```python
from build123d import *

# Parameters (mm, degrees)
SKETCH1_W           = 38.1
SKETCH1_H           = 120.65
SKETCH1_W_2         = 177.8
SKETCH1_H_2         = 177.8
SKETCH1_R           = 14.605
BOSS_EXTRUDE1_DEPTH = 3.175
SKETCH2_R           = 3.175
CUT_EXTRUDE1_DEPTH  = 4.175
SKETCH2_3_W         = 12.7
SKETCH2_3_H         = 38.1
BOSS_EXTRUDE2_DEPTH = 63.5
SKETCH3_R           = 6.35
CUT_EXTRUDE2_DEPTH  = 108.95
CUT_EXTRUDE3_DEPTH  = 4.175


with BuildPart() as part:
    # Sketch1 → Boss-Extrude1 (new body)
    with BuildSketch(Plane.XY):
        with Locations((0, 149.225)):
            Rectangle(SKETCH1_W, SKETCH1_H)
        Rectangle(SKETCH1_W_2, SKETCH1_H_2)
        Circle(SKETCH1_R, mode=Mode.SUBTRACT)
    extrude(amount=BOSS_EXTRUDE1_DEPTH)

    # Sketch2 → Cut-Extrude1 (cut, through all)
    with BuildSketch(Plane.XY.offset(3.175)):
        with Locations((-38.494829198, 22.225)):
            Circle(SKETCH2_R)
        with Locations((38.494829198, 22.225)):
            Circle(SKETCH2_R)
        with Locations((0, -44.45)):
            Circle(SKETCH2_R)
    extrude(amount=-CUT_EXTRUDE1_DEPTH, mode=Mode.SUBTRACT)

    # Sketch2_3 → Boss-Extrude2 (add)
    with BuildSketch(Plane.XY.offset(3.175)):
        with Locations((-12.7, 190.5)):
            Rectangle(SKETCH2_3_W, SKETCH2_3_H)
        with Locations((12.7, 190.5)):
            Rectangle(SKETCH2_3_W, SKETCH2_3_H)
    extrude(amount=BOSS_EXTRUDE2_DEPTH)

    # Sketch3 → Cut-Extrude2 (cut, through all)
    with BuildSketch(Plane.ZY.offset(19.05)):
        with Locations((34.925, 190.5)):
            Circle(SKETCH3_R)
    extrude(amount=-CUT_EXTRUDE2_DEPTH, mode=Mode.SUBTRACT)

    # Sketch4 → Cut-Extrude3 (cut, through all)
    with BuildSketch(Plane.XY.offset(3.175)):
        with BuildLine():
            Line((-19.05, 53.881536726), (-19.05, 88.9))
            Line((-19.05, 88.9), (-88.9, 88.9))
            Line((-88.9, 88.9), (-88.9, -88.9))
            Line((-88.9, -88.9), (88.9, -88.9))
            Line((88.9, -88.9), (88.9, 88.9))
            Line((88.9, 88.9), (19.05, 88.9))
            Line((19.05, 88.9), (19.05, 53.881536726))
            ThreePointArc((19.05, 53.881536726), (46.6627796, 32.995567884), (57.15, 0))
            ThreePointArc((57.15, 0), (-32.995567884, -46.6627796), (-19.05, 53.881536726))
        make_face()
    extrude(amount=-CUT_EXTRUDE3_DEPTH, mode=Mode.SUBTRACT)


solid = part.part
```
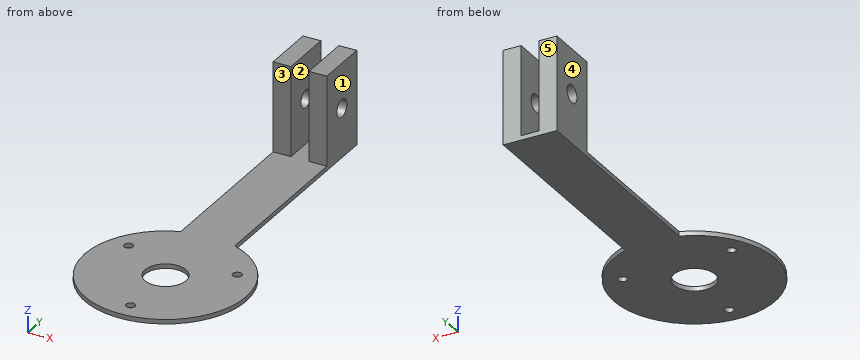
Build history of the part. All positions in model axes, mm. Face numbers are marked on the shaded views. A direction names the side the tool comes from. Coordinates: 2 decimals unless noted, no trailing zeros. Order: outer loops, then holes, each group sorted by start corner. A loop starts at its lowest first (then second) coordinate and runs counter-clockwise, first axis right, second up. Notation, with made-up numbers: (3.25, 87.25) -> (39.25, 87.25) arc R30 ccw to (39.25, 114.25) -> close; hole circle Ø1 at (52, 30). An arc over 180 degrees is marked (long way). Answer in a Markdown table with one row per item. Add a question column.
Q1. Band-saw the part on B-B, the plane x = 0. List the corners of the cut face in (y, z) (3 decimals).
Q2. Which spindle directions (+Z, -Z, +X, -X, +Y, -Y) get a long thin tool onto all of the face, cutting with end or side? Do the marked faces 1, 2, 3, 4 and 5. Say none if no direction does.
Q3. Drop flat-ended pins along their axis: pin 1 (17.5 mm diameter, centred on x = 0, y = 0, fed in from +Z); pin 2 (16.5 mm diameter, centred on y = 190.5, z = 34.925, fed in from -X); pin 3 (6.5 mm diameter, centred on x = 13.5, z = 20, fed in from -Y). Give the stop position or say it passes through.
Q4. Wall check: line 1 along Z through (x, y) = (-15, 53.5) (3 decimals); line 2 along Y through (x, z) = (9.5, 9.5). Give the ranges that are in metal, low to high. Write a range as [from, to].
Q5. Band-saw the part on D-D, the plane y = -44.45. List the corners of the cut face in (x, z) (3 decimals), then the cut area to 3 significant figures.
Q6. Band-saw the part on A-A, the plane y = 190.5. List the corners of the cut face in (x, z) (3 decimals).
Q7. Band-saw the part on C-C, the plane z = 59. List the corners of the cut face in (x, y).
Answers follow:
| question | item | result |
|---|---|---|
| 1 | outline | (-57.15, 0) -> (-47.625, 0) -> (-47.625, 3.175) -> (-57.15, 3.175) -> close; (-41.275, 0) -> (-14.605, 0) -> (-14.605, 3.175) -> (-41.275, 3.175) -> close; (14.605, 0) -> (209.55, 0) -> (209.55, 3.175) -> (14.605, 3.175) -> close |
| 2 | face 1 | +Z, -Z, +X, +Y |
| 2 | face 2 | +Z, +Y, -Y |
| 2 | face 3 | +Z, +X, -X, -Y |
| 2 | face 4 | +Z, -Z, -X, +Y |
| 2 | face 5 | +Z, -Z, +X, -X, +Y |
| 3 | pin 1 | through |
| 3 | pin 2 | x = -19.05 |
| 3 | pin 3 | y = 171.45 |
| 4 | line 1 | [0, 3.175] |
| 4 | line 2 | [171.45, 209.55] |
| 5 | outline | (-35.921, 0) -> (-3.175, 0) -> (-3.175, 3.175) -> (-35.921, 3.175) -> close; (3.175, 0) -> (35.921, 0) -> (35.921, 3.175) -> (3.175, 3.175) -> close |
| 5 | area | 208 mm^2 |
| 6 | outline | (-19.05, 0) -> (19.05, 0) -> (19.05, 28.575) -> (6.35, 28.575) -> (6.35, 3.175) -> (-6.35, 3.175) -> (-6.35, 28.575) -> (-19.05, 28.575) -> close; (-19.05, 41.275) -> (-6.35, 41.275) -> (-6.35, 66.675) -> (-19.05, 66.675) -> close; (6.35, 41.275) -> (19.05, 41.275) -> (19.05, 66.675) -> (6.35, 66.675) -> close |
| 7 | outline | (-19.05, 171.45) -> (-6.35, 171.45) -> (-6.35, 209.55) -> (-19.05, 209.55) -> close; (6.35, 171.45) -> (19.05, 171.45) -> (19.05, 209.55) -> (6.35, 209.55) -> close |
